```python
from build123d import *

# Parameters (mm, degrees)
F2_SIZE = 5.08
F3_SIZE = 2.54


with BuildPart() as f1:
    # F0 (on Front) → F1 (revolve)
    with BuildSketch(Plane.XZ):
        with BuildLine():
            Line((0, 101.6), (0, 127))
            Line((0, 127), (-152.4, 127))
            Line((-152.4, 127), (-152.4, 48.26))
            Line((-152.4, 48.26), (-114.3, 48.26))
            Line((-114.3, 48.26), (-114.3, 79.375))
            ThreePointArc((-114.3, 79.375), (-107.790448, 95.090448), (-92.075, 101.6))
            Line((-92.075, 101.6), (0, 101.6))
        make_face()
    revolve(axis=Axis((-71.717651, 0, 0), (-1, 0, 0)))

    # F2
    f2_edges = [f1.edges().sort_by_distance(p)[0] for p in [
        (-152.4, 0, -127),
    ]]
    chamfer(f2_edges, length=F2_SIZE)

    # F3
    f3_edges = [f1.edges().sort_by_distance(p)[0] for p in [
        (-152.4, 0, -48.26),
        (-114.3, 0, -48.26),
        (-133.35, 0, 48.26),
    ]]
    chamfer(f3_edges, length=F3_SIZE)


solid = f1.part
```
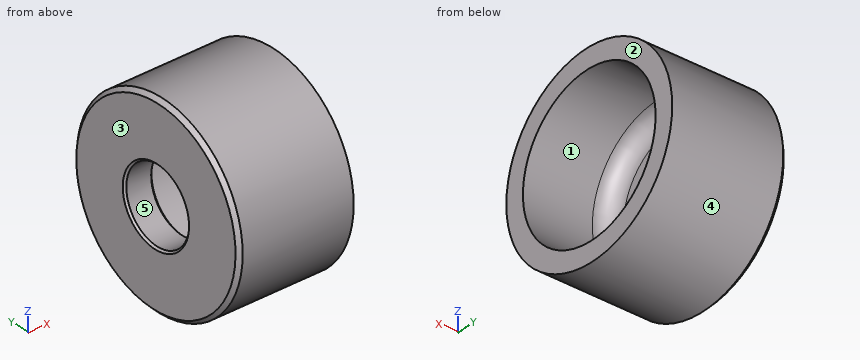
Verification items for the finished model (mm, model axes). Face numbers are marked on the shaded views. A direction names the side the tool comes from. Round coordinates to 2 decimals unless told otherwise and drop trailing zeros. Order: outer loops, then holes, each group sorted by start corner. A loop starts at its lowest first (then second) coordinate and runs counter-clockwise, first axis right, second up.
1) Cross-section at D-D, the plane x = -109. Record the cut outline in (y, z).
Geometry says:
outline: circle Ø254 at (0, 0); hole circle Ø187.56 at (0, 0)
2) Material ranges on line 1 (Y direction, x = -125.5, z = 0); line 2 (Y direction, x = -44, z = 0); line 3 (X direction, y = 59, z = -26.5), recorded low to high.
Geometry says:
line 1: y = -127 to -48.26, 48.26 to 127
line 2: y = -127 to -101.6, 101.6 to 127
line 3: x = -152.4 to -114.3
3) Tool access check on the marked faces 1 and 2. Record the directions out of +Z, -Z, +X, -X, +Y, -Y that give a thin tool (end or side, any length) a straight path to the whole face; none if there is none.
Geometry says:
face 1: +X
face 2: +Z, -Z, +X, +Y, -Y
4) Depth check by flat-ended pin: pin 1 (1.5 mm diameter, centred on x = -133.5, y = 74.5, fed in from +Z); pin 2 (5 mm diameter, centred on x = -18.5, z = -77, fed in from -Y); pin 3 (10 mm diameter, centred on x = -85.5, y = -10, fed in from +Z). Enter the tip coordinate at first touch or a pass-through.
Geometry says:
pin 1: stops at z = 103.39
pin 2: stops at y = -102.85
pin 3: stops at z = 126.9
5) Cross-section at A-A, the plane z = 0. Record the cut outline in (x, y) (3 decimals), plus the area to 3 significant figures.
Geometry says:
outline: (-152.4, -121.92) - (-147.32, -127) - (0, -127) - (0, -101.6) - (-92.075, -101.6) arc R22.225 cw to (-114.3, -79.375) - (-114.3, -50.8) - (-116.84, -48.26) - (-149.86, -48.26) - (-152.4, -50.8) - close; (-152.4, 50.8) - (-149.86, 48.26) - (-116.84, 48.26) - (-114.3, 50.8) - (-114.3, 79.375) arc R22.225 cw to (-92.075, 101.6) - (0, 101.6) - (0, 127) - (-147.32, 127) - (-152.4, 121.92) - close
area: 12,000 mm2
6) Draft check along Y on the marked faces 3, 4 and 5. Enter one of: +Y half, -Y half, draft (parallel to the pull), parting line (faces both ways), or undercut.
Geometry says:
face 3: draft
face 4: parting line
face 5: undercut
7) Cross-section at C-C, the plane x = -15. Record the cut outline in (y, z), plus the area to 3 significant figures.
Geometry says:
outline: circle Ø254 at (0, 0); hole circle Ø203.2 at (0, 0)
area: 18,200 mm2
